Model file for the job. Use its own axes, mm. Round coordinates to 2 decimals unless told otherwise and drop trailing zeros. Loops run counter-clockwise (first coordinate to the right, second up) from the corner with the lowest first, then second, coordinate; pieces in that order, holes last. Notation, with made-up numbers: (65, 0) -> (99, 0) arc R14 cw to (99, 7) -> close; hole circle Ø9 at (69, 14.5). An arc over 180 degrees is marked (long way). Use a Markdown table: item, result. Add a question column.
```python
from build123d import *

# Parameters (mm, degrees)
SKETCH1_W             = 6.7
SKETCH1_H             = 6.7
BOSS_EXTRUDE1_DEPTH   = 1
M3X0_5_TAPPED_HOLE1_D = 2.5
FILLET1_R             = 0.3


with BuildPart() as part:
    # Sketch1 → Boss-Extrude1 (new body)
    with BuildSketch(Plane(origin=(0, 0, 0), x_dir=(1, 0, 0), z_dir=(0, 1, 0))):
        Rectangle(SKETCH1_W, SKETCH1_H)
    extrude(amount=BOSS_EXTRUDE1_DEPTH)

    # M3x0.5 Tapped Hole1 (through all)
    with Locations(Plane(origin=(0, 1, 0), x_dir=(1, 0, 0), z_dir=(0, 1, 0))):
        with Locations((0, 0)):
            Hole(M3X0_5_TAPPED_HOLE1_D / 2)

    # Fillet1
    fillet1_edges = [part.edges().sort_by_distance(p)[0] for p in [
        (3.35, 0.5, 3.35),
        (-3.35, 0.5, 3.35),
        (-3.35, 0.5, -3.35),
        (3.35, 0.5, -3.35),
    ]]
    fillet(fillet1_edges, radius=FILLET1_R)


solid = part.part
```
1) Wall check: probe 1 along Z at (x, y) = (0, 0.65); probe 2 along Z at (x, y) = (0.5, 0.7); probe 3 along X at (y, z) = (0.9, 0.25). Give the ranges that are in metal, low to high. Write a range as from..to.
2) Cut at C-C on y = 0.5. Write the cut outline in (x, z), and give its area (3 significant figures).
3) Cut at B-B on x = 0. Write the cut outline in (y, z), and give its area (3 significant figures).
4) Cut at A-A on z = -0.75. Write the cut outline in (x, y).
5) Pull direction Z, two halves, no side cores. Call faces 1 (the face through (0, 0.5, 3.35)), 2 (the face through (-2, 1, 0)), 3 (the face through (0.27, 0.49, 1.22)): +Z half, -Z half, draft (parallel to the pull), parting line (faces both ways), or undercut.
Established:
| question | item | result |
|---|---|---|
| 1 | probe 1 | z = -3.35..-1.25, 1.25..3.35 |
| 1 | probe 2 | z = -3.35..-1.15, 1.15..3.35 |
| 1 | probe 3 | x = -3.35..-1.22, 1.22..3.35 |
| 2 | outline | (-3.35, -3.05) arc R0.3 ccw to (-3.05, -3.35) -> (3.05, -3.35) arc R0.3 ccw to (3.35, -3.05) -> (3.35, 3.05) arc R0.3 ccw to (3.05, 3.35) -> (-3.05, 3.35) arc R0.3 ccw to (-3.35, 3.05) -> close; hole circle Ø2.5 at (0, 0) |
| 2 | area | 39.9 mm^2 |
| 3 | outline | (0, -3.35) -> (1, -3.35) -> (1, -1.25) -> (0, -1.25) -> close; (0, 1.25) -> (1, 1.25) -> (1, 3.35) -> (0, 3.35) -> close |
| 3 | area | 4.20 mm^2 |
| 4 | outline | (-3.35, 0) -> (-1, 0) -> (-1, 1) -> (-3.35, 1) -> close; (1, 0) -> (3.35, 0) -> (3.35, 1) -> (1, 1) -> close |
| 5 | face 1 | +Z half |
| 5 | face 2 | draft |
| 5 | face 3 | undercut |
